For this review, take the finished solid that the model builds, in its own axes (mm). Give positions to 0.01 mm unless a question says otherwise; leave off trailing zeros. Write each loop counter-clockwise with the first axis right and the second up, starting at its lowest first coordinate (ties: lowest second). Pieces come first, ordered by that corner, then holes. Notation, with made-up numbers: M 32,34.5 L 74,34.5 A20 cw 74,61.5 Z; hole C -24,59.5 d2. An arc over 180 degrees is marked long. Write item = value, one per line.
```python
from build123d import *

# Parameters (mm, degrees)
SKETCH14_R            = 5
BOSS_EXTRUDE1_DEPTH   = 160
BOSS_EXTRUDE1_2_DEPTH = 160
SKETCH15_W            = 160
SKETCH15_H            = 40
BOSS_EXTRUDE2_DEPTH   = 3
LPATTERN1_COUNT       = 30
LPATTERN1_PITCH       = 10.931034483


with BuildPart() as part:
    # Sketch14 → Boss-Extrude1 (new, symmetric)
    with BuildSketch(Plane(origin=(0, 0, 0), x_dir=(1, 0, 0), z_dir=(0, 1, 0))):
        with Locations(Location((-40, 0, 0), (0, 0, 270))):
            Circle(SKETCH14_R)
    extrude(amount=BOSS_EXTRUDE1_DEPTH, both=True)



with BuildPart() as body_2:
    # Sketch14 → Boss-Extrude1 2 (new, symmetric)
    with BuildSketch(Plane(origin=(0, 0, 0), x_dir=(1, 0, 0), z_dir=(0, 1, 0))):
        with Locations(Location((40, 0, 0), (0, 0, 270))):
            Circle(SKETCH14_R)
    extrude(amount=BOSS_EXTRUDE1_2_DEPTH, both=True)


with BuildPart() as part_1:
    add(part.part)

    add(body_2.part)  # Boss-Extrude2 merges body 2
    # Sketch15 → Boss-Extrude2 (add)
    with BuildSketch(Plane(origin=(0, 160, 0), x_dir=(1, 0, 0), z_dir=(0, 1, 0))):
        Rectangle(SKETCH15_W, SKETCH15_H)
    boss_extrude2 = extrude(amount=-BOSS_EXTRUDE2_DEPTH)

    # LPattern1: Boss-Extrude2 ×30
    with Locations(*[(0, -i * LPATTERN1_PITCH, 0) for i in range(1, LPATTERN1_COUNT)]):
        add(boss_extrude2)


solid = part_1.part
```
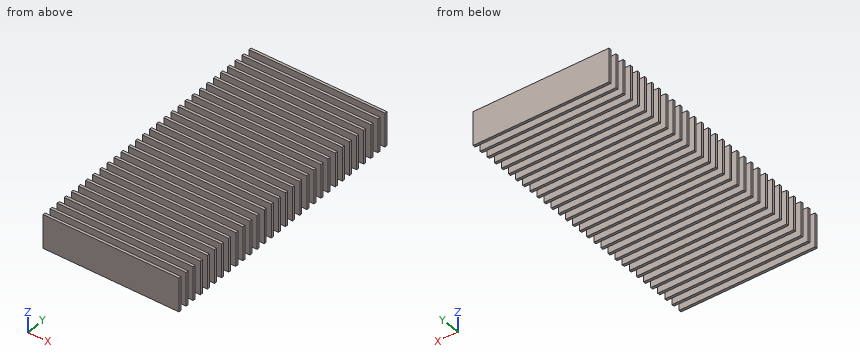
1. We need section B-B, the plane y = 98. Write out the cut boundary in (x, z).
Responses:
outline = C -40,0 d10; C 40,0 d10
2. We need section A-A, the plane z = 16.5. Count the separate pieces of the cut face and the enclosed holes in it, then the cut area to 3 significant figures.
Responses:
separate_pieces = 30
enclosed_holes = 0
area = 14,400 mm2
3. Insertion check: P1, Ø1.5, axis at y = -52, z = -15.5, coming from the +X side. The pin has a flat end and moves straight along its axis. Give the tip position at first contact, or say it passes through.
Responses:
P1 = through
4. For line 1 along X through (y, z) = (-8, -3.5); line 2 along X through (y, z) = (-30, 3); line 3 along Z through (x, y) = (41, 121), list the stretches that pass through material, from the lowest coordinate up. Write a range as from..to.
Responses:
line_1 = -43.57..-36.43, 36.43..43.57
line_2 = -44..-36, 36..44
line_3 = -4.9..4.9
